```python
from build123d import *

# Parameters (mm, degrees)
BOSS_EXTRUDE1_DEPTH = 25
SKETCH2_R           = 50
BOSS_EXTRUDE2_DEPTH = 25
SKETCH3_R           = 25
CUT_EXTRUDE2_DEPTH  = 25


with BuildPart() as part:
    # Sketch1 → Boss-Extrude1 (new body)
    with BuildSketch(Plane.XY):
        with BuildLine():
            ThreePointArc((-500, 100), (-600, 0), (-500, -100))
            ThreePointArc((-500, -100), (0, -68.626966597), (500, -100))
            ThreePointArc((500, -100), (600, 0), (500, 100))
            ThreePointArc((500, 100), (0, 68.626966597), (-500, 100))
        make_face()
    extrude(amount=BOSS_EXTRUDE1_DEPTH)

    # Sketch2 → Boss-Extrude2 (add)
    with BuildSketch(Plane(origin=(0, 0, 0), x_dir=(1, 0, 0), z_dir=(0, 0, -1))):
        with Locations((-500, 0)):
            Circle(SKETCH2_R)
    extrude(amount=BOSS_EXTRUDE2_DEPTH)

    # Sketch3 → Cut-Extrude2 (cut)
    with BuildSketch(Plane.XY.offset(25)):
        with Locations((500, 0)):
            Circle(SKETCH3_R)
    extrude(amount=-CUT_EXTRUDE2_DEPTH, mode=Mode.SUBTRACT)


solid = part.part
```
Source: CAD feature listing. Evaluate the final solid. Frame: model axes, mm. Coordinates: 2 decimals unless noted, no trailing zeros. Loops run counter-clockwise (first coordinate to the right, second up) from the corner with the lowest first, then second, coordinate; pieces in that order, holes last. Notation, with made-up numbers: (-37, 22.5) - (-12, 22.5) arc R31 cw to (-12, 46.5) - close; hole circle Ø8 at (57, -33.75). An arc over 180 degrees is marked (long way). Answer as CSV lines item,"result".
1. Section B-B (z = 15.5). Return loops of the section in (x, y), then the cut area to 3 significant figures.
Established:
outline,"(-500, -100) arc R4000 cw to (500, -100) arc R100 ccw to (500, 100) arc R4000 cw to (-500, 100) arc R100 ccw to start; hole circle Ø50 at (500, 0)"
area,"188,000 mm2"
2. Section A-A (y = 0). Return loops of the section in (x, z).
Established:
outline,"(-600, 0) - (-550, 0) - (-550, -25) - (-450, -25) - (-450, 0) - (475, 0) - (475, 25) - (-600, 25) - close; (525, 0) - (600, 0) - (600, 25) - (525, 25) - close"
3. Section D-D (x = 318). Return loops of the section in (y, z).
Established:
outline,"(-81.29, 0) - (81.29, 0) - (81.29, 25) - (-81.29, 25) - close"
4. Ray query, line 1 (Z direction, x = 245, y = -21); line 2 (Y direction, x = -276, z = 18); line 3 (X direction, y = 10, z = -22). Return the intervals inside material, ascending.
Established:
line 1,"z = 0 to 25"
line 2,"y = -78.16 to 78.16"
line 3,"x = -548.99 to -451.01"
5. Section C-C (x = -275.5). Return loops of the section in (y, z).
Established:
outline,"(-78.13, 0) - (78.13, 0) - (78.13, 25) - (-78.13, 25) - close"
6. Contact query for flat-ended pins moving along their axis: pin 1 (1 mm diameter, centred on y = 7.5, z = -15.5, fed in from +X); pin 2 (1 mm diameter, centred on y = 14.5, z = -19.5, fed in from -X); pin 3 (12 mm diameter, centred on x = -433.5, y = -18, fed in from -Z). Output: stop coordinate, or through.
Established:
pin 1,"stops at x = -450.49"
pin 2,"stops at x = -548"
pin 3,"stops at z = 0"
7. Mould query, pull axis X, two halves, no side actions, for faces 1 (the cylindrical face through (-7.018, -68.633, 12.325)), 2 (the cylindrical face through (-452.31, -15.02, -12.32)), 3 (the cylindrical face through (-599.976, 2.199, 12.325)). Classes: released by +X, released by -X, zero draft, split by the parting line, or undercut.
Established:
face 1,"undercut"
face 2,"split by the parting line"
face 3,"released by -X"
